Source: CAD feature listing. Evaluate the final solid. Frame: model axes, mm. A direction names the side the tool comes from. Coordinates: 2 decimals unless noted, no trailing zeros. Loops run counter-clockwise (first coordinate to the right, second up) from the corner with the lowest first, then second, coordinate; pieces in that order, holes last.
```python
from build123d import *

# Parameters (mm, degrees)
CHAMFER_1_SIZE           = 2
HOLE_WIZARD_M3_1_D       = 3
CUT_EXTRUDE_1_DEPTH      = 97.046863561
CUT_EXTRUDE_1_DEPTH_BACK = 97.046863561
HOLE_WIZARD_M3_1_2_D     = 2.5


with BuildPart() as part:
    # 草图1 → 旋转1 (revolve)
    with BuildSketch(Plane(origin=(0, 0, 0), x_dir=(0, 0, -1), z_dir=(1, 0, 0))):
        Polygon((32, 0), (50, 0), (50, 5), (35, 5), (35, 65), (16, 65), (16, 60), (32, 60), align=None)
    revolve(axis=Axis((0, 0, 0), (0, 1, 0)))

    # 倒角1
    chamfer_1_edges = [part.edges().sort_by_distance(p)[0] for p in [
        (0, 65, 16),
    ]]
    chamfer(chamfer_1_edges, length=CHAMFER_1_SIZE)

    # Hole Wizard M3 _1 (through all)
    with Locations(Plane(origin=(0, 65, 0), x_dir=(1, 0, 0), z_dir=(0, 1, 0))):
        with Locations((19, -13), (-19, 13), (-19, -13), (19, 13)):
            Hole(HOLE_WIZARD_M3_1_D / 2)

    # 草图4 → 切除-拉伸1 (cut, two sides: drawn at the far end of the back side and taken through both)
    with BuildSketch(Plane(origin=(0, 0, 0), x_dir=(0, 0, -1), z_dir=(1, 0, 0)).offset(-CUT_EXTRUDE_1_DEPTH_BACK)):
        with BuildLine():
            Line((-14, 10), (14, 10))
            ThreePointArc((14, 10), (18.242640687, 11.757359313), (20, 16))
            Line((20, 16), (20, 44))
            ThreePointArc((20, 44), (18.242640687, 48.242640687), (14, 50))
            Line((14, 50), (-14, 50))
            ThreePointArc((-14, 50), (-18.242640687, 48.242640687), (-20, 44))
            Line((-20, 44), (-20, 16))
            ThreePointArc((-20, 16), (-18.242640687, 11.757359313), (-14, 10))
        make_face()
    extrude(amount=CUT_EXTRUDE_1_DEPTH + CUT_EXTRUDE_1_DEPTH_BACK, mode=Mode.SUBTRACT)

    # Hole Wizard M3 _1 2 (through all)
    with Locations(Plane(origin=(0, 0, 0), x_dir=(-1, 0, 0), z_dir=(0, -1, 0))):
        with Locations((47, 0), (23.5, -40.703193978), (-23.5, -40.703193978), (-47, 0), (-23.5, 40.703193978), (23.5, 40.703193978)):
            Hole(HOLE_WIZARD_M3_1_2_D / 2)


solid = part.part
```
Q1. Section query C-C on x = 23.5. Return the cut outline in (y, z), then the cut area to 3 significant figures.
Q2. Draft query along X for faces 4 (the cylindrical face through (-1.41, 29.58, 31.97)), 5 (the cylindrical face through (-15.02, 2.54, -47.69)), 6 (the flat face through (33, 10, 0)). Return one class per face: released by +X, released by -X, zero draft, split by the parting line, or undercut.
Q3. Section query B-B on x = 0. Return the cut outline in (y, z).
Q4. First-contact query: pin 1 Ø1 at (x, y) = (-12.5, 53) entering from -Z; pin 2 Ø5 at (y, z) = (49, 17) entering from -X; pin 3 Ø12 at (x, z) = (19, 40) entering from +Y. Flat tips, straight axial feed; report the tip coordinate or a pass-through.
Q5. Material intervals for line 1 along Z through (x, y) = (-23.5, 3.85); line 2 along Z through (x, y) = (-19, 63.85); line 3 along X through (y, z) = (62.1, -13), sorted ascending.
Q6. Section query A-A on y = 31.5. Return the cut outline in (x, z).
Q7. Section query D-D on z = -5. Count the separate pieces of the cut face and the enclosed holes in it, then the cut area to 3 significant figures.
Q8. Reachability of faces 1 (the flat face through (33, 0, -1)), 2 (the flat face through (-27, 30, 20)), 3 (the cylindrical face through (-1.539, 35.42, 34.966)) from +Z, -Z, +X, -X, +Y, -Y: full face, straight path, thin tool, end or side. Return the list, or none.
Resolved:
1. outline: (0, -44.13) - (5, -44.13) - (5, -41.95) - (0, -41.95) - close; (0, -39.45) - (5, -39.45) - (5, -25.94) - (65, -25.94) - (65, 25.94) - (5, 25.94) - (5, 39.45) - (0, 39.45) - (0, 21.72) - (60, 21.72) - (60, -21.72) - (0, -21.72) - close; (0, 41.95) - (5, 41.95) - (5, 44.13) - (0, 44.13) - close
1. area: 922 mm2
2. face 4: undercut
2. face 5: split by the parting line
2. face 6: zero draft
3. outline: (0, -50) - (5, -50) - (5, -35) - (65, -35) - (65, -18) - (63, -16) - (60, -16) - (60, -32) - (0, -32) - close; (0, 32) - (60, 32) - (60, 16) - (63, 16) - (65, 18) - (65, 35) - (5, 35) - (5, 50) - (0, 50) - close
4. pin 1: stops at z = -32.88
4. pin 2: stops at x = -31.77
4. pin 3: stops at y = 5
5. line 1: z = -44.13 to -41.95, -39.45 to -21.72, 21.72 to 39.45, 41.95 to 44.13
5. line 2: z = -29.39 to -14.5, -11.5 to 11.5, 14.5 to 29.39
5. line 3: x = -32.5 to -20.5, -17.5 to -9.33, 9.33 to 17.5, 20.5 to 32.5
6. outline: (-28.72, -20) arc R35 ccw to (28.72, -20) - (24.98, -20) arc R32 cw to (-24.98, -20) - close; (-28.72, 20) - (-24.98, 20) arc R32 cw to (24.98, 20) - (28.72, 20) arc R35 ccw to start
7. separate pieces: 4
7. enclosed holes: 0
7. area: 463 mm2
8. face 1: +Z, -Z, +X, -X, -Y
8. face 2: +X, -X
8. face 3: +Y
